```python
from build123d import *

# Parameters (mm, degrees)
SKETCH1_R               = 5
SKETCH1_R_2             = 4
BOSS_EXTRUDE1_DEPTH     = 16.1
CHAMFER1_SIZE           = 0.2
CHAMFER2_SIZE           = 0.363970234
CHAMFER2_SIZE_2         = 1
CUT_EXTRUDE1_REACH      = 21.557
CUT_EXTRUDE1_END_RADIUS = 4
SKETCH2_R               = 1.5
CIRPATTERN1_COUNT       = 2
CIRPATTERN1_ANGLE       = 90


with BuildPart() as part:
    # Sketch1 → Boss-Extrude1 (new body)
    with BuildSketch(Plane(origin=(0, 0, 0), x_dir=(1, 0, 0), z_dir=(0, 1, 0))):
        with Locations(Location((0, 0, 0), (0, 0, 270))):
            Circle(SKETCH1_R)
        with Locations(Location((0, 0, 0), (0, 0, 270))):
            Circle(SKETCH1_R_2, mode=Mode.SUBTRACT)
    extrude(amount=BOSS_EXTRUDE1_DEPTH)

    # Chamfer1
    chamfer1_edges = [part.edges().sort_by_distance(p)[0] for p in [
        (0, 0, -5),
        (0, 0, -4),
        (0, 16.1, -4),
    ]]
    chamfer(chamfer1_edges, length=CHAMFER1_SIZE)

    # Chamfer2
    # the kernel refuses this chamfer: 1, 0.363970234 mm, written as the material it takes off along each edge
    with BuildSketch(Plane(origin=(0, 16.1, 0), x_dir=(0, 0, 1), z_dir=(-1, 0, 0))) as chamfer2_piece_1:
        Polygon((5, -CHAMFER2_SIZE), (5 - CHAMFER2_SIZE_2, 0), (5, 0), align=None)
    revolve(axis=Axis((0, 16.1, 0), (0, 1, 0)), mode=Mode.SUBTRACT)

    # Cut-Extrude1: up to this cylinder (the profile starts outside it)
    cut_extrude1_end = Plane(origin=(0, 3.5, 0), z_dir=(0, -1, 0)) * Cylinder(CUT_EXTRUDE1_END_RADIUS, 52.114, mode=Mode.PRIVATE)
    # Sketch2 → Cut-Extrude1 (cut, up to the surface)
    with BuildSketch(Plane(origin=(0, 0, -5), x_dir=(-1, 0, 0), z_dir=(0, 0, -1)), mode=Mode.PRIVATE) as cut_extrude1_sk1:
        with Locations((0, 3.5)):
            Circle(SKETCH2_R)
    cut_extrude1_tool1 = extrude(cut_extrude1_sk1.sketch, amount=-CUT_EXTRUDE1_REACH, mode=Mode.PRIVATE) - cut_extrude1_end
    cut_extrude1 = cut_extrude1_tool1.solids().sort_by_distance((0, 3.5, -5))[0]
    add(cut_extrude1, mode=Mode.SUBTRACT)

    # CirPattern1: Cut-Extrude1 ×2 about axis
    cirpattern1_axis = Axis((0, 15.9, 0), (0, -1, 0))
    for i in range(1, CIRPATTERN1_COUNT):
        add(cut_extrude1.rotate(cirpattern1_axis, i * CIRPATTERN1_ANGLE / (CIRPATTERN1_COUNT - 1)), mode=Mode.SUBTRACT)


solid = part.part
```
The model under review builds one solid part; all positions refer to its coordinate system, in mm. A direction names the side the tool comes from. Give positions to 0.01 mm unless a question says otherwise; leave off trailing zeros. Order: outer loops, then holes, each group sorted by start corner. A loop starts at its lowest first (then second) coordinate and runs counter-clockwise, first axis right, second up. Notation, with made-up numbers: (79.25, 36) - (113.25, 36) arc R27 cw to (113.25, 60) - close; hole circle Ø4 at (10.25, 15). An arc over 180 degrees is marked (long way). Use CSV: the item, a comma, the result in double quotes. Start each with the question number.
Q1. We need section B-B, the plane x = 0. Write out the cut boundary in (y, z).
Q2. To check wall thickness, follow line 1 along Z through (x, y) = (0, 11.5); line 2 along Z through (x, y) = (0.75, 2); line 3 along X through (y, z) = (1, -2). State the ranges of each line that lie inside material, in increasing order. Write a range as [from, to].
Q3. Tool access review of faces 3 (the cylindrical face through (-4.436, 7.859, 2.307)), 4 (the cylindrical face through (4.363, 2.925, -1.386)): name each direction out of +Z, -Z, +X, -X, +Y, -Y from which nothing blocks a thin tool from reaching the whole face with its end or side.
Q4. We need section A-A, the plane z = 0. Write out the cut boundary in (x, y), and give its area (3 significant figures).
Q5. Clearance check with a flat-ended pin moving along its axis: pin 1 Ø4 at (x, y) = (3, 3) entering from +Z. State where the tip first meets the part, or that it passes through.
Q6. The part is to be moulded in two halves that separate along Y. For faces 1 (the cylindrical face through (-1.386, 2.925, -4.363)), 2 (the flat face through (-4, 0, 2)), say which applies: +Y half, -Y half, draft (parallel to the pull), parting line (faces both ways), or undercut.
Q7. We need section D-D, the plane y = 10.5. Write out the cut boundary in (x, z), and give its area (3 significant figures).
Q8. We need section C-C, the plane y = 3.5. Write out the cut boundary in (x, z).
Outcome:
1,outline,"(0, -4.8) - (0.2, -5) - (2, -5) - (2, -4) - (0.2, -4) - (0, -4.2) - close; (0, 4.2) - (0.2, 4) - (15.9, 4) - (16.05, 4.15) - (15.74, 5) - (0.2, 5) - (0, 4.8) - close; (5, -5) - (15.74, -5) - (16.05, -4.15) - (15.9, -4) - (5, -4) - close"
2,line 1,"z = [-5, -4], [4, 5]"
2,line 2,"z = [-4.94, -3.93], [3.93, 4.94]"
2,line 3,"x = [-4.58, -3.46], [3.46, 4.58]"
3,face 3,"+Y, -Y"
3,face 4,"+X"
4,outline,"(-5, 0.2) - (-4.8, 0) - (-4.2, 0) - (-4, 0.2) - (-4, 15.9) - (-4.15, 16.05) - (-5, 15.74) - close; (4, 0.2) - (4.2, 0) - (4.8, 0) - (5, 0.2) - (5, 2) - (4, 2) - close; (4, 5) - (5, 5) - (5, 15.74) - (4.15, 16.05) - (4, 15.9) - close"
4,area,"28.7 mm^2"
5,pin 1,"stops at z = 4.9"
6,face 1,"undercut"
6,face 2,"-Y half"
7,outline,"circle Ø10 at (0, 0); hole circle Ø8 at (0, 0)"
7,area,"28.3 mm^2"
8,outline,"(-1.5, -4.77) - (-1.5, -3.71) arc R4 cw (long way) to (3.71, 1.5) - (4.77, 1.5) arc R5 ccw (long way) to start; (1.5, -4.77) arc R5 ccw to (4.77, -1.5) - (3.71, -1.5) arc R4 cw to (1.5, -3.71) - close"
